Geometry check sheet. Reference: the model listing, model coordinates, mm. Round coordinates to 2 decimals unless told otherwise and drop trailing zeros. Write each loop counter-clockwise with the first axis right and the second up, starting at its lowest first coordinate (ties: lowest second). Pieces come first, ordered by that corner, then holes.
Item 1: Depth check by flat-ended pin: P1, Ø1.2, axis at x = 51, y = 2.5, coming from the +Z side; P2, Ø1.2, axis at y = 2, z = 31, coming from the -X side; P3, Ø1, axis at x = 22.5, y = 1.5, coming from the +Z side; P4, Ø24, axis at x = 25, z = 0, coming from the +Y side. Enter the tip coordinate at first touch or a pass-through.
Item 2: Cross-section at D-D (z = 21.5). Enter the section's corners in (x, y).
Item 3: Cross-section at C-C (y = 1.05). Enter the section's corners in (x, z), then the cut area to 3 significant figures.
Item 4: Cross-section at B-B (x = 25). Enter the section's corners in (y, z), then the cut area to 3 significant figures.
Item 5: Cross-section at A-A (z = 0). Enter the section's corners in (x, y).
Item 6: Scan lines: probe 1 along X at (y, z) = (2.05, 0); probe 2 along Z at (x, y) = (25, 2); probe 3 along X at (y, z) = (2.1, 11.5). Record each from-to range of solid material in increasing order.
Autodesk Inventor part; units mm, degrees
ref_plane "YZ Plane" through (0, 0, 0) normal (1, 0, 0) x (0, 1, 0)
ref_plane "XZ Plane" through (0, 0, 0) normal (0, 1, 0) x (-1, 0, 0)
ref_plane "XY Plane" through (0, 0, 0) normal (0, 0, 1) x (1, 0, 0)
sketch "Sketch1" plane through (0, 0, 0) normal (0, 1, 0) x (-1, 0, 0)
  line L0 (50, 30) -> (-50, 30) construction
  line L1 (-50, 30) -> (-50, -30) construction
  line L2 (-50, -30) -> (50, -30) construction
  line L3 (50, -30) -> (50, 30) construction
  line L4 (20, 30) -> (-20, 30) construction
  line L5 (-20, 30) -> (-20, 34)
  line L6 (-20, 34) -> (20, 34)
  line L7 (20, 34) -> (20, 30)
  line L8 (20, -30) -> (-20, -30) construction
  line L9 (-20, -30) -> (-20, -34)
  line L10 (-20, -34) -> (20, -34)
  line L11 (20, -34) -> (20, -30)
  line L12 (-50, -20) -> (-54, -20)
  line L13 (-54, -20) -> (-54, 20)
  line L14 (-54, 20) -> (-50, 20)
  line L15 (-50, 20) -> (-50, -20) construction
  line L16 (50, -20) -> (54, -20)
  line L17 (54, -20) -> (54, 20)
  line L18 (54, 20) -> (50, 20)
  line L19 (50, 20) -> (50, -20) construction
  line L20 (50, -20) -> (50, -30)
  line L21 (50, -30) -> (20, -30)
  line L22 (-20, -30) -> (-50, -30)
  line L23 (-50, -20) -> (-50, -30)
  line L24 (-50, 20) -> (-50, 30)
  line L25 (-20, 30) -> (-50, 30)
  line L26 (50, 20) -> (50, 30)
  line L27 (50, 30) -> (20, 30)
  point P0 (0, 0)
  point P1 (52, -20)
  point P2 (-52, 20)
  point P3 (52, 20)
  point P4 (0, -30)
  point P5 (0, 30)
  point P6 (50, 0)
  point P7 (-50, 0)
  point P8 (0, -30)
  point P9 (50, 0)
  dimension "d0" = 40
  dimension "d1" = 4
  dimension "d2" = 100
  dimension "d3" = 60
extrude "Extrusion1" add sketch "Sketch1" along normal blind 4
sketch "Sketch2" plane through (0, 4, 0) normal (0, 1, 0) x (1, 0, 0)
  circle A0 centre (25, 0) radius 15
  line L0 (50, 20) -> (50, 30)
  point P0 (0, 0)
  dimension "d6" = 30
  dimension "d7" = 10
extrude "Extrusion2" cut sketch "Sketch2" against normal blind 4
properties part number "SideMale_100wx60h_V1" material "Wood (Oak)"
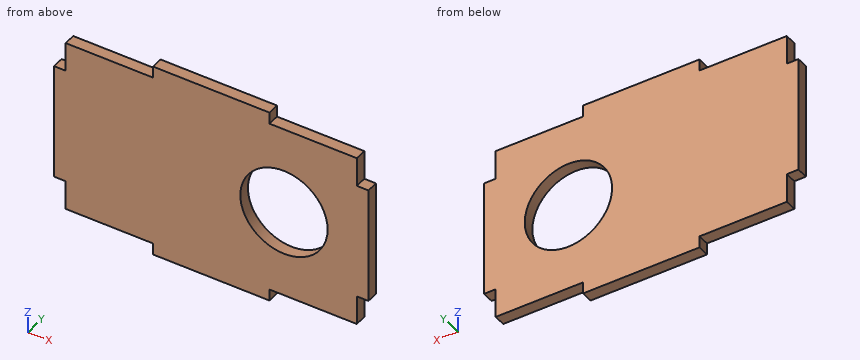
Resolved:
1. P1: stops at z = 20
1. P2: stops at x = -20
1. P3: stops at z = 30
1. P4: passes through
2. outline: (-50, 0) - (50, 0) - (50, 4) - (-50, 4) - close
3. outline: (-54, -20) - (-50, -20) - (-50, -30) - (-20, -30) - (-20, -34) - (20, -34) - (20, -30) - (50, -30) - (50, -20) - (54, -20) - (54, 20) - (50, 20) - (50, 30) - (20, 30) - (20, 34) - (-20, 34) - (-20, 30) - (-50, 30) - (-50, 20) - (-54, 20) - close; hole circle Ø30 at (25, 0)
3. area: 5,930 mm2
4. outline: (0, -30) - (4, -30) - (4, -15) - (0, -15) - close; (0, 15) - (4, 15) - (4, 30) - (0, 30) - close
4. area: 120 mm2
5. outline: (-54, 0) - (10, 0) - (10, 4) - (-54, 4) - close; (40, 0) - (54, 0) - (54, 4) - (40, 4) - close
6. probe 1: x = -54 to 10, 40 to 54
6. probe 2: z = -30 to -15, 15 to 30
6. probe 3: x = -54 to 15.37, 34.63 to 54
